Design review of the part built by this model. Coordinates are the model's own, in mm. Coordinates: 2 decimals unless noted, no trailing zeros. Write each loop counter-clockwise with the first axis right and the second up, starting at its lowest first coordinate (ties: lowest second). Pieces come first, ordered by that corner, then holes.
Q1. To check wall thickness, follow probe 1 along Y at (x, z) = (25.4, 1.1); probe 2 along Y at (x, z) = (25, 0.55). State the ranges of each line that lie inside material, in increasing order.
Q2. The part is to be moulded in two halves that separate along Y. For faces 1 (the face through (0, 25.4, 1)), 2 (the face through (26.83, 22.04, 0.76)), 3 (the face through (29.21, 0, 1)), say which applies: +Y half, -Y half, draft (parallel to the pull), parting line (faces both ways), or undercut.
Q3. Add section B-B, the plane y = -21.59. Give the boundary of the cut face in (x, z).
Q4. Add section A-A, the plane x = -25.4. Give the boundary of the cut face in (y, z), plus the area to 3 significant figures.
from build123d import *

# Parameters (mm, degrees)
SKETCH_W     = 58.42
SKETCH_H     = 50.8
PAD_DEPTH    = 1.5
SKETCH001_R  = 1.5
POCKET_DEPTH = 5


with BuildPart() as part:
    # Sketch → Pad (new body)
    with BuildSketch(Plane.XY):
        Rectangle(SKETCH_W, SKETCH_H)
    extrude(amount=PAD_DEPTH)

    # Sketch001 → Pocket (cut)
    with BuildSketch(Plane.XY.offset(1.5)):
        with Locations((-25.4, 21.59)):
            Circle(SKETCH001_R)
        with Locations((25.4, 21.59)):
            Circle(SKETCH001_R)
        with Locations((25.4, -21.59)):
            Circle(SKETCH001_R)
        with Locations((-25.4, -21.59)):
            Circle(SKETCH001_R)
    extrude(amount=-POCKET_DEPTH, mode=Mode.SUBTRACT)


solid = part.part
Here are the results:
1. probe 1: y = -25.4 to -23.09, -20.09 to 20.09, 23.09 to 25.4
1. probe 2: y = -25.4 to -23.04, -20.14 to 20.14, 23.04 to 25.4
2. face 1: +Y half
2. face 2: undercut
2. face 3: draft
3. outline: (-29.21, 0) - (-26.9, 0) - (-26.9, 1.5) - (-29.21, 1.5) - close; (-23.9, 0) - (23.9, 0) - (23.9, 1.5) - (-23.9, 1.5) - close; (26.9, 0) - (29.21, 0) - (29.21, 1.5) - (26.9, 1.5) - close
4. outline: (-25.4, 0) - (-23.09, 0) - (-23.09, 1.5) - (-25.4, 1.5) - close; (-20.09, 0) - (20.09, 0) - (20.09, 1.5) - (-20.09, 1.5) - close; (23.09, 0) - (25.4, 0) - (25.4, 1.5) - (23.09, 1.5) - close
4. area: 67.2 mm2
